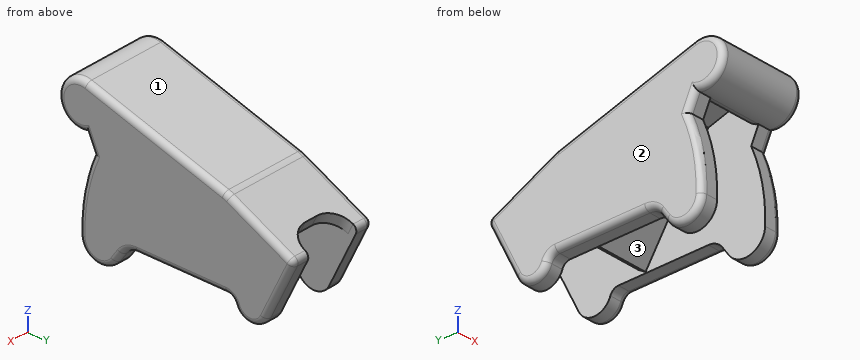
from build123d import *

# Parameters (mm, degrees)
PAD004_DEPTH    = 7.65
POCKET003_DEPTH = 4.65
POCKET004_DEPTH = 2
FILLET007_R     = 1
FILLET008_R     = 1


with BuildPart() as part:
    # Sketch009 → Pad004 (new body, symmetric)
    with BuildSketch(Plane.YZ):
        with BuildLine():
            ThreePointArc((-2.8284271247, -1), (-0.1735950846, -2.9949732464), (2.6939497909, -1.3200888318))
            Line((2.6939497909, -1.3200888318), (7.8, 9.1))
            Line((7.8, 9.1), (-3.7, 14.7352281014))
            ThreePointArc((-3.7, 14.7352281014), (-4.158961759, 14.9368094594), (-4.6331484619, 15.0993760945))
            Line((-4.6331484619, 15.0993760945), (-28.6904310189, 22.2388309237))
            ThreePointArc((-28.6904310189, 22.2388309237), (-33.6993372116, 18.5718979166), (-28.8290152057, 14.7228067922))
            Line((-27.5290152057, 11.9228067922), (-28.8290152057, 14.7228067922))
            ThreePointArc((-27.5290152057, 11.9228067922), (-29.4749197629, 5.5883007232), (-29.9826934773, -1.0188679245))
            ThreePointArc((-29.9826934773, -1.0188679245), (-27.4803397166, -4.255402597), (-23.6176804166, -2.9075175272))
            Line((-23.6176804166, -2.9075175272), (-22.4775697078, -1.2792706909))
            ThreePointArc((-20.0201135749, 0), (-21.4053594146, -0.3389675005), (-22.4775697078, -1.2792706909))
            Line((-4.2426406871, 0), (-20.0201135749, 0))
            ThreePointArc((-2.8284271247, -1), (-3.3766152833, -0.2752551286), (-4.2426406871, 0))
        make_face()
    extrude(amount=PAD004_DEPTH, both=True)

    # Sketch010 → Pocket003 (cut, symmetric)
    with BuildSketch(Plane.YZ):
        with BuildLine():
            Line((6.9199407788, 7.3040334727), (-5.8060355253, 13.5400142802))
            ThreePointArc((-5.8060355253, 13.5400142802), (-11.1364622888, 12.5033421393), (-11.5881769744, 7.0918642957))
            Line((-11.5881769744, 7.0918642957), (-7.7326639328, 1.0024084327))
            Line((-9, 0.2), (-7.7326639328, 1.0024084327))
            Line((-9, 0.2), (-20, 17.5735670895))
            Line((-24.6418524264, 18.9511248267), (-20, 17.5735670895))
            ThreePointArc((-24.6418524264, 18.9511248267), (-25.4821110434, 18.8237971917), (-25.9209782539, 18.0960318164))
            ThreePointArc((-28.8290152057, 14.7228067922), (-26.8461376765, 15.9534931036), (-25.9209782539, 18.0960318164))
            Line((-28.8290152057, 14.7228067922), (-34.6400816793, 13.2289840317))
            Line((-34.6400816793, 13.2289840317), (-31.0800592212, -4.6959665273))
            Line((-31.0800592212, -4.6959665273), (6.9199407788, -4.6959665273))
            Line((6.9199407788, -4.6959665273), (6.9199407788, 7.3040334727))
        make_face()
    extrude(amount=POCKET003_DEPTH, both=True, mode=Mode.SUBTRACT)

    # Sketch011 (on Face6 of Pocket003) → Pocket004 (cut)
    with BuildSketch(Plane(origin=(0, 5.1060502091, 10.4200888318), x_dir=(0, -0.8979832636, 0.4400296106), z_dir=(0, 0.4400296106, 0.8979832636))):
        with BuildLine():
            Line((-3, 4.65), (-2, 4.65))
            ThreePointArc((1.5, 1.15), (0.4748737342, 3.6248737342), (-2, 4.65))
            Line((1.5, 1.15), (1.5, -1.15))
            ThreePointArc((-2, -4.65), (0.4748737342, -3.6248737342), (1.5, -1.15))
            Line((-2, -4.65), (-3, -4.65))
            Line((-3, -4.65), (-3, 4.65))
        make_face()
    extrude(amount=-POCKET004_DEPTH, mode=Mode.SUBTRACT)

    # Fillet007
    fillet007_edges = [part.edges().sort_by_distance(p)[0] for p in [
        (-6.15, 7.8, 9.1),
        (6.15, 7.8, 9.1),
    ]]
    fillet(fillet007_edges, radius=FILLET007_R)

    # Fillet008
    fillet008_edges = [part.edges().sort_by_distance(p)[0] for p in [
        (7.65, -16.66179, 18.669104),
        (-7.65, -16.66179, 18.669104),
        (-7.65, -28.179015, 13.322807),
        (7.65, -28.179015, 13.322807),
    ]]
    fillet(fillet008_edges, radius=FILLET008_R)


with BuildPart() as part_1:
    # Body003 placement: moved
    add(part.part.moved(Location((0, 15.2, 5.2))))


solid = part_1.part
Design review of the part built by this model. Coordinates are the model's own, in mm. Face numbers are marked on the shaded views. Coordinates: 2 decimals unless noted, no trailing zeros. Order: outer loops, then holes, each group sorted by start corner. A loop starts at its lowest first (then second) coordinate and runs counter-clockwise, first axis right, second up.
Item 1: For line 1 (X direction, y = 19, z = 12.5); line 2 (Y direction, x = -4, z = 14.5); line 3 (Z direction, x = 0.75, y = 5.5), list the stretches that pass through material, from the lowest coordinate up.
Item 2: Take a section at A-A, the plane x = 4. Write out the cut boundary in (y, z), then the cut area to 3 significant figures.
Item 3: The part is to be moulded in two halves that separate along X. For the marked faces 1, 2 and 3, say which applies: pulls with the +X half, pulls with the -X half, needs draft (parallel to the pull), parting line crosses it, or undercut.
Item 4: For pin 1 Ø2 at (x, y) = (-6, -0.5) entering from -Z; pin 2 Ø1.5 at (x, z) = (1, 12) entering from -Y; pin 3 Ø4 at (x, y) = (0, -4) entering from -Z, all flat-tipped, find the tip position at first contact; note any pin that passes through.
The answers:
1. line 1: x = -7.65 to -4.65, 4.65 to 7.65
1. line 2: y = 0.44 to 2.92, 18.05 to 19.72
1. line 3: z = 6.51 to 9.31, 18.77 to 21.8
2. outline: (-13.49, 27.44) arc R3.9 ccw (long way) to (-10.72, 23.3) arc R1 cw to (-9.44, 24.15) - (-4.8, 22.77) - (6.2, 5.4) - (7.47, 6.2) - (3.61, 12.29) arc R4.5 cw to (9.39, 18.74) - (19.4, 13.84) - (20.28, 15.63) - (11.5, 19.94) arc R6 ccw to (10.57, 20.3) - close
2. area: 171 mm2
3. face 1: needs draft
3. face 2: pulls with the -X half
3. face 3: undercut
4. pin 1: stops at z = 5.2
4. pin 2: stops at y = 1.55
4. pin 3: stops at z = 18.35
